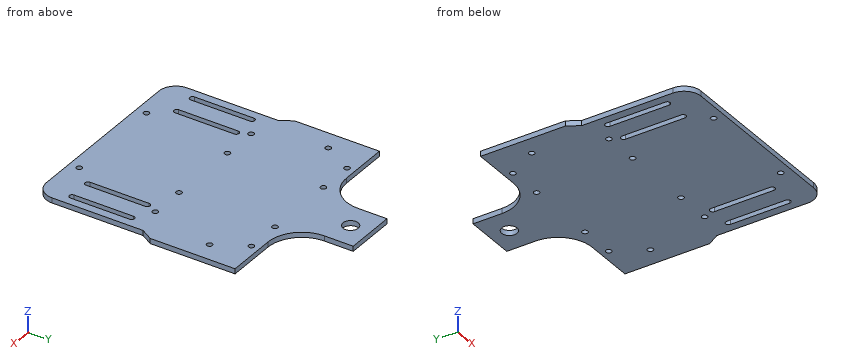
from build123d import *

# Parameters (mm, degrees)
SKETCH1_R           = 4.5
SKETCH1_R_2         = 1.65
BOSS_EXTRUDE1_DEPTH = 3
FILLET3_R           = 20
FILLET4_R           = 10


with BuildPart() as part:
    # Sketch1 → Boss-Extrude1 (new body)
    with BuildSketch(Plane.XY):
        Polygon((402.495772407, 1683.241435849), (402.495772407, 1633.241435849), (406.628072987, 1626.391319652), (406.628072987, 1562.767892621), (526.628072987, 1562.767892621), (526.628072987, 1626.391319652), (530.760373568, 1633.241435849), (530.760373568, 1683.241435849), (481.628072987, 1683.241435849), (481.628072987, 1720.241435849), (451.628072987, 1720.241435849), (451.628072987, 1683.241435849), align=None)
        with Locations((466.628072987, 1708.767892621)):
            Circle(SKETCH1_R, mode=Mode.SUBTRACT)
        with Locations((519.320878863, 1660.655786173)):
            Circle(SKETCH1_R_2, mode=Mode.SUBTRACT)
        with Locations((496.449751686, 1568.767892621)):
            Circle(SKETCH1_R_2, mode=Mode.SUBTRACT)
        with Locations(Location((413.935267112, 1660.655786173, 0), (0, 0, 180))):
            Circle(SKETCH1_R_2, mode=Mode.SUBTRACT)
        with Locations(Location((436.806394289, 1568.767892621, 0), (0, 0, 180))):
            Circle(SKETCH1_R_2, mode=Mode.SUBTRACT)
        with Locations((488.128072987, 1678.491435849)):
            Circle(SKETCH1_R_2, mode=Mode.SUBTRACT)
        with Locations(Location((509.128072987, 1678.491435849, 0), (0, 0, 180))):
            Circle(SKETCH1_R_2, mode=Mode.SUBTRACT)
        with Locations(Location((488.128072987, 1621.991435849, 0), (0, 0, 180))):
            Circle(SKETCH1_R_2, mode=Mode.SUBTRACT)
        with Locations((509.128072987, 1621.991435849)):
            Circle(SKETCH1_R_2, mode=Mode.SUBTRACT)
        with Locations(Location((424.128072987, 1621.991435849, 0), (0, 0, 180))):
            Circle(SKETCH1_R_2, mode=Mode.SUBTRACT)
        with Locations((424.128072987, 1678.491435849)):
            Circle(SKETCH1_R_2, mode=Mode.SUBTRACT)
        with Locations(Location((445.128072987, 1678.491435849, 0), (0, 0, 180))):
            Circle(SKETCH1_R_2, mode=Mode.SUBTRACT)
        with Locations((445.128072987, 1621.991435849)):
            Circle(SKETCH1_R_2, mode=Mode.SUBTRACT)
        with BuildLine():
            Line((414.778072987, 1615.267892621), (414.778072987, 1580.267892621))
            ThreePointArc((414.778072987, 1580.267892621), (413.128072987, 1578.617892621), (411.478072987, 1580.267892621))
            Line((411.478072987, 1580.267892621), (411.478072987, 1615.267892621))
            ThreePointArc((411.478072987, 1615.267892621), (413.128072987, 1616.917892621), (414.778072987, 1615.267892621))
        make_face(mode=Mode.SUBTRACT)
        with BuildLine():
            Line((518.478072987, 1615.267892621), (518.478072987, 1580.267892621))
            ThreePointArc((518.478072987, 1580.267892621), (520.128072987, 1578.617892621), (521.778072987, 1580.267892621))
            Line((521.778072987, 1580.267892621), (521.778072987, 1615.267892621))
            ThreePointArc((521.778072987, 1615.267892621), (520.128072987, 1616.917892621), (518.478072987, 1615.267892621))
        make_face(mode=Mode.SUBTRACT)
        with BuildLine():
            Line((428.778072987, 1615.267892621), (428.778072987, 1580.267892621))
            ThreePointArc((428.778072987, 1580.267892621), (427.128072987, 1578.617892621), (425.478072987, 1580.267892621))
            Line((425.478072987, 1580.267892621), (425.478072987, 1615.267892621))
            ThreePointArc((425.478072987, 1615.267892621), (427.128072987, 1616.917892621), (428.778072987, 1615.267892621))
        make_face(mode=Mode.SUBTRACT)
        with BuildLine():
            Line((504.478072987, 1615.267892621), (504.478072987, 1580.267892621))
            ThreePointArc((504.478072987, 1580.267892621), (506.128072987, 1578.617892621), (507.778072987, 1580.267892621))
            Line((507.778072987, 1580.267892621), (507.778072987, 1615.267892621))
            ThreePointArc((507.778072987, 1615.267892621), (506.128072987, 1616.917892621), (504.478072987, 1615.267892621))
        make_face(mode=Mode.SUBTRACT)
    extrude(amount=BOSS_EXTRUDE1_DEPTH)

    # Fillet3
    fillet3_edges = [part.edges().sort_by_distance(p)[0] for p in [
        (481.628072987, 1683.241435849, 1.5),
        (451.628072987, 1683.241435849, 1.5),
    ]]
    fillet(fillet3_edges, radius=FILLET3_R)

    # Fillet4
    fillet4_edges = [part.edges().sort_by_distance(p)[0] for p in [
        (526.628072987, 1562.767892621, 1.5),
        (406.628072987, 1562.767892621, 1.5),
    ]]
    fillet(fillet4_edges, radius=FILLET4_R)


solid = part.part
For this review, take the finished solid that the model builds, in its own axes (mm). Give positions to 0.01 mm unless a question says otherwise; leave off trailing zeros. Loops run counter-clockwise (first coordinate to the right, second up) from the corner with the lowest first, then second, coordinate; pieces in that order, holes last. Notation, with made-up numbers: M 76,-1.5 L 84,-1.5 A17 ccw 84,2.5 Z; hole C 88.5,29.5 d2. An arc over 180 degrees is marked long. Answer as a JSON object with one key per item and string values. Group by question number.
Q1. Add section B-B on z = 2. Give the number of separate pieces and of enclosed holes in the cut face, and give its area (3 significant figures).
Q2. Add section D-D on y = 1687.5. Give the boundary of the cut face in (x, z).
Q3. Add section C-C on y = 1575. Give the boundary of the cut face in (x, z), and give its area (3 significant figures).
Q4. Add section A-A on y = 1601.5. Give the boundary of the cut face in (x, z), and give its area (3 significant figures).
Q5. Insertion check: P1, Ø2.5, axis at x = 496.45, y = 1568.77, coming from the -Z side; P2, Ø1.5, axis at y = 1603.5, z = 2, coming from the +X side; P3, Ø1.5, axis at x = 519.5, z = 1.5, coming from the +Y side; P4, Ø1.5, axis at y = 1626.5, z = 1.5, coming from the +X side. Each pin has a flat end and moves straight along its axis. Give the tip position at first contact, or say it passes through.
Q6. For probe 1 along X at (y, z) = (1608, 0.8); probe 2 along Y at (x, z) = (509, 2.8); probe 3 along Y at (x, z) = (519.5, 1.4), list the stretches that pass through material, from the lowest coordinate up. Write a range as [from, to].
Checked values:
{
 "1": {"separate pieces": "1", "enclosed holes": "17", "area": "15,500 mm²"},
 "2": {"outline": "M 443.97,0 L 489.29,0 L 489.29,3 L 443.97,3 Z"},
 "3": {"outline": "M 406.63,0 L 526.63,0 L 526.63,3 L 406.63,3 Z", "area": "360 mm²"},
 "4": {"outline": "M 406.63,0 L 411.48,0 L 411.48,3 L 406.63,3 Z; M 414.78,0 L 425.48,0 L 425.48,3 L 414.78,3 Z; M 428.78,0 L 504.48,0 L 504.48,3 L 428.78,3 Z; M 507.78,0 L 518.48,0 L 518.48,3 L 507.78,3 Z; M 521.78,0 L 526.63,0 L 526.63,3 L 521.78,3 Z", "area": "320 mm²"},
 "5": {"P1": "through", "P2": "x = 526.63", "P3": "y = 1683.24", "P4": "x = 527.15"},
 "6": {"probe 1": "[406.63, 411.48], [414.78, 425.48], [428.78, 504.48], [507.78, 518.48], [521.78, 526.63]", "probe 2": "[1562.77, 1620.35], [1623.64, 1676.85], [1680.14, 1683.24]", "probe 3": "[1563.19, 1578.74], [1616.79, 1659.02], [1662.3, 1683.24]"}
}
